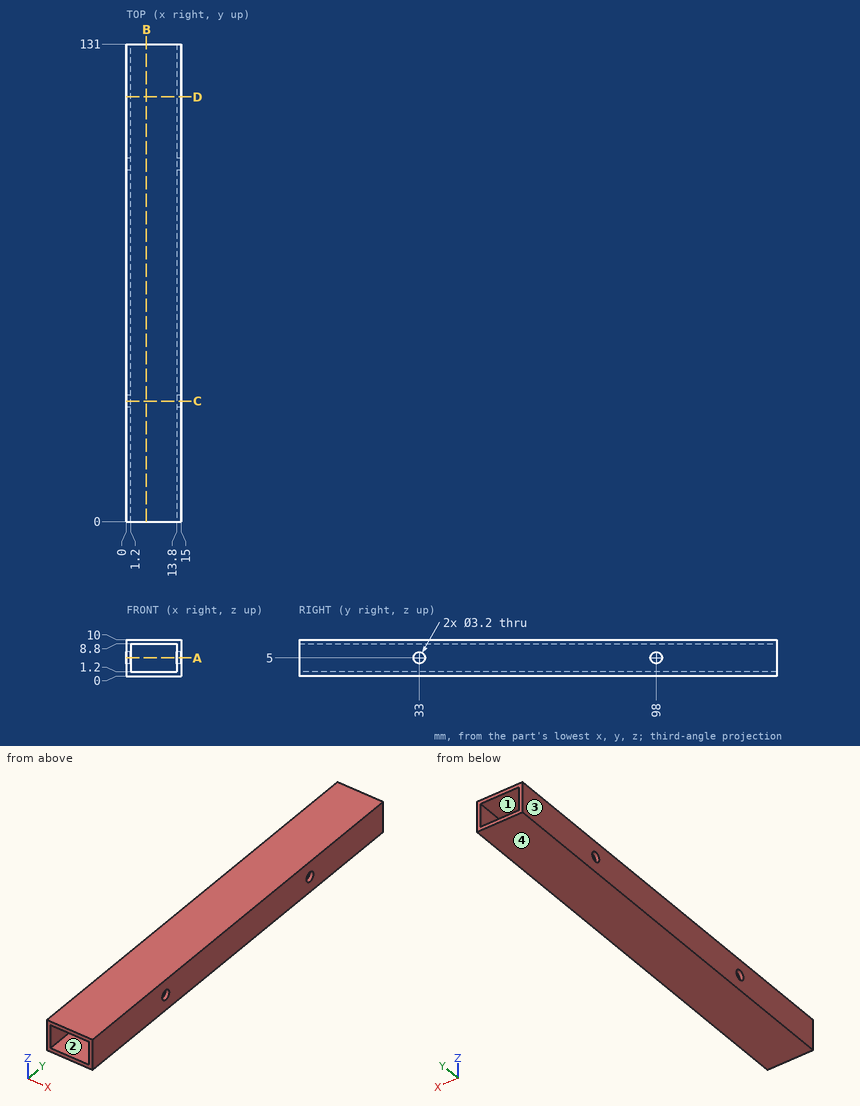
Input: dimensioned drawing with shaded views. Units: mm. Origin: part minimum x, y, z. Give positions to 0.01 mm unless a question says otherwise; leave off trailing zeros. Write each loop counter-clockwise with the first axis right and the second up, starting at its lowest first coordinate (ties: lowest second). Pieces come first, ordered by that corner, then holes. Notation, with made-up numbers: M 86.25,8.25 L 109.25,8.25 A19 ccw 109.25,34.25 Z; hole C 12.25,86.5 d2. An arc over 180 degrees is marked long. Return JSON: item names as keys, results as strings. Group by question number.
1) Cut plane B-B, the plane x = 5.5. Output: boundary loops of the cut face in (y, z), plus the area to 3 significant figures.
2) Pull-direction query (Z, two-part tool) for the marked faces 1, 2, 3 and 4; classes: pulls with the +Z half, pulls with the -Z half, needs draft (parallel to the pull), parting line crosses it, or undercut.
3) Cut plane A-A, the plane z = 5. Output: boundary loops of the cut face in (x, y), plus the area to 3 significant figures.
4) Pin query (flat end, axial travel): P1, Ø3, axis at y = 33, z = 5, coming from the -X side. Return the tip coordinate at first contact, or that it passes through.
5) Cut plane C-C, the plane y = 33. Output: boundary loops of the cut face in (x, z), plus the area to 3 significant figures.
6) Cut plane D-D, the plane y = 116.5. Output: boundary loops of the cut face in (x, z), plus the area to 3 significant figures.
7) Material intervals for line 1 along Y through (x, z) = (0.75, 5); line 2 along Z through (x, y) = (0.7, 98); line 3 along X through (y, z) = (36.5, 4.25), sorted ascending. Write a range as [from, to].
Recorded:
{
 "1": {"outline": "M 0,0 L 131,0 L 131,1.2 L 0,1.2 Z; M 0,8.8 L 131,8.8 L 131,10 L 0,10 Z", "area": "314 mm²"},
 "2": {"face 1": "undercut", "face 2": "undercut", "face 3": "needs draft", "face 4": "pulls with the -Z half"},
 "3": {"outline": "M 0,0 L 1.2,0 L 1.2,31.4 L 0,31.4 Z; M 0,34.6 L 1.2,34.6 L 1.2,96.4 L 0,96.4 Z; M 0,99.6 L 1.2,99.6 L 1.2,131 L 0,131 Z; M 13.8,0 L 15,0 L 15,31.4 L 13.8,31.4 Z; M 13.8,34.6 L 15,34.6 L 15,96.4 L 13.8,96.4 Z; M 13.8,99.6 L 15,99.6 L 15,131 L 13.8,131 Z", "area": "299 mm²"},
 "4": {"P1": "passes through"},
 "5": {"outline": "M 0,0 L 15,0 L 15,3.4 L 13.8,3.4 L 13.8,1.2 L 1.2,1.2 L 1.2,3.4 L 0,3.4 Z; M 0,6.6 L 1.2,6.6 L 1.2,8.8 L 13.8,8.8 L 13.8,6.6 L 15,6.6 L 15,10 L 0,10 Z", "area": "46.6 mm²"},
 "6": {"outline": "M 0,0 L 15,0 L 15,10 L 0,10 Z; hole M 1.2,1.2 L 13.8,1.2 L 13.8,8.8 L 1.2,8.8 Z", "area": "54.2 mm²"},
 "7": {"line 1": "y = [0, 31.4], [34.6, 96.4], [99.6, 131]", "line 2": "z = [0, 3.4], [6.6, 10]", "line 3": "x = [0, 1.2], [13.8, 15]"}
}
